Here's how the part is built. I have some questions about the finished solid (model axes, mm). A direction names the side the tool comes from. Give positions to 0.01 mm unless a question says otherwise; leave off trailing zeros. Order: outer loops, then holes, each group sorted by start corner. A loop starts at its lowest first (then second) coordinate and runs counter-clockwise, first axis right, second up.
from build123d import *

# Parameters (mm, degrees)
F0_R     = 7.9375
F0_R_2   = 12.7
F0_R_3   = 6.35
F1_DEPTH = 12.7
F2_DEPTH = 25.4


with BuildPart() as f1:
    # F0 (on Front) → F1 (new body)
    with BuildSketch(Plane.XZ):
        with BuildLine():
            Line((82.55, 7.45639), (82.55, 34.925))
            ThreePointArc((82.55, 34.925), (50.896024, 66.674855), (19.050581, 35.117047))
            ThreePointArc((19.050581, 35.117047), (18.051201, 32.734953), (15.663106, 31.75))
            Line((15.663106, 31.75), (0, 31.75))
            Line((0, 31.75), (-15.663106, 31.75))
            ThreePointArc((-15.663106, 31.75), (-18.051201, 32.734953), (-19.050581, 35.117047))
            ThreePointArc((-19.050581, 35.117047), (-50.896024, 66.674855), (-82.55, 34.925))
            Line((-82.55, 34.925), (-82.55, 7.45639))
            ThreePointArc((-82.55, 7.45639), (-83.623483, 4.44432), (-86.36, 2.790112))
            ThreePointArc((-86.36, 2.790112), (-101.503534, -17.789696), (-82.55, -34.925))
            Line((-82.55, -34.925), (-53.975, -34.925))
            ThreePointArc((-53.975, -34.925), (-47.239808, -37.714808), (-44.45, -44.45))
            Line((-44.45, -44.45), (-44.45, -41.275))
            ThreePointArc((-44.45, -41.275), (-38.870384, -54.745384), (-25.4, -60.325))
            Line((-25.4, -60.325), (-19.05, -60.325))
            Line((-19.05, -60.325), (-19.05, -51.58833))
            ThreePointArc((-19.05, -51.58833), (0, -32.53833), (19.05, -51.58833))
            Line((19.05, -51.58833), (19.05, -60.325))
            Line((19.05, -60.325), (25.4, -60.325))
            ThreePointArc((25.4, -60.325), (38.870384, -54.745384), (44.45, -41.275))
            Line((44.45, -41.275), (44.45, -44.45))
            ThreePointArc((44.45, -44.45), (47.239808, -37.714808), (53.975, -34.925))
            Line((53.975, -34.925), (82.55, -34.925))
            ThreePointArc((82.55, -34.925), (101.503534, -17.789696), (86.36, 2.790112))
            ThreePointArc((86.36, 2.790112), (83.623483, 4.44432), (82.55, 7.45639))
        make_face()
        with Locations((-82.55, -15.875)):
            Circle(F0_R, mode=Mode.SUBTRACT)
        Circle(F0_R_2, mode=Mode.SUBTRACT)
        with Locations((82.55, -15.875)):
            Circle(F0_R, mode=Mode.SUBTRACT)
        with Locations((-50.8, 34.925)):
            Circle(F0_R_2, mode=Mode.SUBTRACT)
        with Locations((50.8, 34.925)):
            Circle(F0_R_2, mode=Mode.SUBTRACT)
        with Locations((-82.55, -15.875)):
            Circle(F0_R)
        with Locations((-82.55, -15.875)):
            Circle(F0_R_3, mode=Mode.SUBTRACT)
        with Locations((82.55, -15.875)):
            Circle(F0_R)
        with Locations((82.55, -15.875)):
            Circle(F0_R_3, mode=Mode.SUBTRACT)
    extrude(amount=F1_DEPTH)

    # F0 (on Front) → F2 (join)
    with BuildSketch(Plane.XZ):
        with Locations((82.55, -15.875)):
            Circle(F0_R)
        with Locations((82.55, -15.875)):
            Circle(F0_R_3, mode=Mode.SUBTRACT)
        with Locations((-82.55, -15.875)):
            Circle(F0_R)
        with Locations((-82.55, -15.875)):
            Circle(F0_R_3, mode=Mode.SUBTRACT)
    extrude(amount=-F2_DEPTH)


solid = f1.part
Q1. If we section it at B-B on z = 40: List the corners of the cut face in (x, y) for me, plus the area to 3 significant figures.
Filled sheet:
outline: (-82.14, -12.7) - (-62.44, -12.7) - (-62.44, 0) - (-82.14, 0) - close; (-39.16, -12.7) - (-19.46, -12.7) - (-19.46, 0) - (-39.16, 0) - close; (19.46, -12.7) - (39.16, -12.7) - (39.16, 0) - (19.46, 0) - close; (62.44, -12.7) - (82.14, -12.7) - (82.14, 0) - (62.44, 0) - close
area: 1,000 mm2
Q2. I need wall thicknesses on L1, parallel to Z at x = 83, y = 18; L2, parallel to X at y = -8, z = -20.5; L3, parallel to X at y = 2, z = -15. Which ranges of each line are inside material? Lowest first, please.
Filled sheet:
L1: z = -23.8 to -22.21, -9.54 to -7.95
L2: x = -101.03 to -86.9, -78.2 to 78.2, 86.9 to 101.03
L3: x = -90.44 to -88.84, -76.26 to -74.66, 74.66 to 76.26, 88.84 to 90.44
Q3. For faces 4 (the face through (-82.55, -6, 21)), 5 (the face through (68, -6, -34.925)), 6 (the face through (-78.89, 12.52, -22.92)), which set-ups out of +Z, -Z, +X, -X, +Y, -Y let a thin tool reach every point of the face, with its end or its side?
Filled sheet:
face 4: +Z, -X, +Y, -Y
face 5: -Z, +X, +Y, -Y
face 6: +Y
Q4. I'm going to push flat-ended pins straight in: P1, Ø4.5, axis at y = -3.5, z = -58, coming from the -X side; P2, Ø10, axis at y = 2.5, z = 37.5, coming from the -X side; P3, Ø10, axis at x = 39, z = 0, coming from the +Y side. Where does each tip first touch, or does it pass through?
Filled sheet:
P1: stops at x = -37.78
P2: stops at x = -82.55
P3: stops at y = 0
Q5. Thinking about a two-plate mould opening in Z: for faces 1 (the face through (-2.75, -6.26, -12.4)), 2 (the face through (-50.2, -6.26, 66.67)), 3 (the face through (101.46, -6.26, -18.18)), which applies, released by +Z, released by -Z, zero draft, split by the parting line, or undercut?
Filled sheet:
face 1: undercut
face 2: released by +Z
face 3: split by the parting line
Q6. If we section it at A-A on x = -50.8: List the corners of the cut face in (y, z) for me (3 decimals), plus the area to 3 significant figures.
Filled sheet:
outline: (-12.7, -35.47) - (0, -35.47) - (0, 22.225) - (-12.7, 22.225) - close; (-12.7, 47.625) - (0, 47.625) - (0, 66.675) - (-12.7, 66.675) - close
area: 975 mm2
Q7. If we section it at D-D on z = -38: List the corners of the cut face in (x, y) for me, plus the area to 3 significant figures.
Filled sheet:
outline: (-46.97, -12.7) - (-13.35, -12.7) - (-13.35, 0) - (-46.97, 0) - close; (13.35, -12.7) - (46.97, -12.7) - (46.97, 0) - (13.35, 0) - close
area: 854 mm2
Q8. If we section it at C-C on y = 8.5: Give the number of separate pieces and of enclosed holes in the cut face, plus the area to 3 significant figures.
Filled sheet:
separate pieces: 2
enclosed holes: 2
area: 143 mm2
